```python
from build123d import *

# Parameters (mm, degrees)
F0_R     = 13.725453
F1_DEPTH = 7


with BuildPart() as f1:
    # F0 (on Top) → F1 (new body)
    with BuildSketch(Plane.XY):
        with BuildLine():
            Line((5, 43.660253), (-5, 43.660253))
            Line((-5, 43.660253), (-7.886752, 43.660253))
            Line((-7.886752, 43.660253), (-9.330152, 41.160211))
            Line((-9.330152, 41.160211), (-14.330019, 32.500187))
            Line((-14.330019, 32.500187), (-15.773503, 30))
            ThreePointArc((-15.773503, 30), (-14.879368, 28.590608), (-14.105865, 27.111568))
            ThreePointArc((-14.105865, 27.111568), (-14.879368, 8.590607), (-30.53224, -1.339746))
            ThreePointArc((-30.53224, -1.339746), (-32.199876, -1.409392), (-33.867513, -1.339746))
            Line((-33.867513, -1.339746), (-35.310889, -3.839746))
            Line((-35.310889, -3.839746), (-40.310889, -12.5))
            Line((-40.310889, -12.5), (-41.754264, -15))
            Line((-41.754264, -15), (-40.310888, -17.499999))
            Line((-40.310888, -17.499999), (-35.310888, -26.160254))
            Line((-35.310888, -26.160254), (-33.867512, -28.660255))
            Line((-33.867512, -28.660255), (-30.980762, -28.660255))
            Line((-30.980762, -28.660255), (-20.980762, -28.660255))
            Line((-20.980762, -28.660255), (-18.094012, -28.660255))
            ThreePointArc((-18.094012, -28.660255), (-17.320508, -27.181214), (-16.426373, -25.77182))
            ThreePointArc((-16.426373, -25.77182), (0, -17.181214), (16.426373, -25.77182))
            ThreePointArc((16.426373, -25.77182), (17.320508, -27.181214), (18.094012, -28.660255))
            Line((18.094012, -28.660255), (20.980762, -28.660255))
            Line((20.980762, -28.660255), (30.980762, -28.660255))
            Line((30.980762, -28.660255), (33.867512, -28.660255))
            Line((33.867512, -28.660255), (35.310888, -26.160254))
            Line((35.310888, -26.160254), (40.309298, -17.502755))
            Line((40.309298, -17.502755), (41.754264, -15))
            Line((41.754264, -15), (40.310625, -12.499543))
            Line((40.310625, -12.499543), (35.312513, -3.84256))
            Line((35.312513, -3.84256), (33.867513, -1.339746))
            ThreePointArc((33.867513, -1.339746), (32.199876, -1.409392), (30.53224, -1.339746))
            ThreePointArc((30.53224, -1.339746), (14.879368, 8.590607), (14.105865, 27.111568))
            ThreePointArc((14.105865, 27.111568), (14.879368, 28.590608), (15.773503, 30))
            Line((15.773503, 30), (14.329358, 32.501332))
            Line((14.329358, 32.501332), (9.330202, 41.160124))
            Line((9.330202, 41.160124), (7.886752, 43.660253))
            Line((7.886752, 43.660253), (5, 43.660253))
        make_face()
        Polygon((-30.980762, -6.339746), (-20.980762, -6.339746), (-15.980762, -15), (-20.980762, -23.660254), (-30.980762, -23.660254), (-35.980762, -15), align=None, mode=Mode.SUBTRACT)
        Circle(F0_R, mode=Mode.SUBTRACT)
        Polygon((20.980762, -23.660254), (15.980762, -15), (20.980762, -6.339746), (30.980762, -6.339746), (35.980762, -15), (30.980762, -23.660254), align=None, mode=Mode.SUBTRACT)
        Polygon((10, 30), (5, 21.339746), (-5, 21.339746), (-10, 30), (-5, 38.660254), (5, 38.660254), align=None, mode=Mode.SUBTRACT)
    extrude(amount=F1_DEPTH)


solid = f1.part
```
The model under review builds one solid part; all positions refer to its coordinate system, in mm. A direction names the side the tool comes from. Round coordinates to 2 decimals unless told otherwise and drop trailing zeros. Loops run counter-clockwise (first coordinate to the right, second up) from the corner with the lowest first, then second, coordinate; pieces in that order, holes last. Notation, with made-up numbers: (83.25, -2.75) -> (96.25, -2.75) arc R16 cw to (96.25, 12.25) -> close; hole circle Ø8 at (5.5, 1). An arc over 180 degrees is marked (long way). Answer in a Markdown table with one row per item.
1) Consider section C-C, the plane y = -19.5. Write out the cut boundary in (x, z), plus the area to 3 significant figures.
Taken from the geometry:
| item | result |
|---|---|
| outline | (-39.16, 0) -> (-33.38, 0) -> (-33.38, 7) -> (-39.16, 7) -> close; (-18.58, 0) -> (-9.35, 0) -> (-9.35, 7) -> (-18.58, 7) -> close; (9.35, 0) -> (18.58, 0) -> (18.58, 7) -> (9.35, 7) -> close; (33.38, 0) -> (39.16, 0) -> (39.16, 7) -> (33.38, 7) -> close |
| area | 210 mm² |
2) Consider section B-B, the plane y = 0. Write out the cut boundary in (x, z), plus the area to 3 significant figures.
Taken from the geometry:
| item | result |
|---|---|
| outline | (-24.82, 0) -> (-13.73, 0) -> (-13.73, 7) -> (-24.82, 7) -> close; (13.73, 0) -> (24.82, 0) -> (24.82, 7) -> (13.73, 7) -> close |
| area | 155 mm² |
3) Consider section A-A, the plane x = 0. Write out the cut boundary in (y, z), plus the area to 3 significant figures.
Taken from the geometry:
| item | result |
|---|---|
| outline | (-17.18, 0) -> (-13.73, 0) -> (-13.73, 7) -> (-17.18, 7) -> close; (13.73, 0) -> (21.34, 0) -> (21.34, 7) -> (13.73, 7) -> close; (38.66, 0) -> (43.66, 0) -> (43.66, 7) -> (38.66, 7) -> close |
| area | 112 mm² |
4) For pin 1 Ø2 at (y, z) = (12, 1) entering from -X; pin 2 Ø1.5 at (y, z) = (-9.5, 3.5) entering from -X; pin 3 Ø8 at (x, y) = (-21, 33.5) entering from -Z; pin 4 Ø2 at (x, z) = (-24, 4) entering from +Y, all flat-tipped, find the tip position at first contact; note any pin that passes through.
Taken from the geometry:
| item | result |
|---|---|
| pin 1 | stops at x = -13.7 |
| pin 2 | stops at x = -39.01 |
| pin 3 | passes through |
| pin 4 | stops at y = 0.83 |
5) Tool access review of faces 1 (the cylindrical face through (-14.89, 28.61, 3.45)), 2 (the cylindrical face through (-17.33, -27.2, 3.45)), 3 (the flat face through (-26, -6.34, 3)), 4 (the cylindrical face through (14.868, 28.57, 3.451)): name each direction out of +Z, -Z, +X, -X, +Y, -Y from which nothing blocks a thin tool from reaching the whole face with its end or side.
Taken from the geometry:
| item | result |
|---|---|
| face 1 | +Z, -Z, -X |
| face 2 | +Z, -Z, -Y |
| face 3 | +Z, -Z |
| face 4 | +Z, -Z, +X |
6) Consider section D-D, the plane x = 11. Write out the cut boundary in (y, z).
Taken from the geometry:
| item | result |
|---|---|
| outline | (-20.48, 0) -> (-8.21, 0) -> (-8.21, 7) -> (-20.48, 7) -> close; (8.21, 0) -> (38.27, 0) -> (38.27, 7) -> (8.21, 7) -> close |
7) Wall thickness on line 1 along Y through (x, z) = (0, 5); line 2 along Y through (x, z) = (7.5, 6.75); line 3 along X through (y, z) = (-11.5, 2.75): over which ranges is each line inside the solid? List them lowest first.
Taken from the geometry:
| item | result |
|---|---|
| line 1 | y = -17.18 to -13.73, 13.73 to 21.34, 38.66 to 43.66 |
| line 2 | y = -18.64 to -11.5, 11.5 to 25.67, 34.33 to 43.66 |
| line 3 | x = -39.73 to -33.96, -18 to -7.49, 7.49 to 18, 33.96 to 39.73 |
